For this review, take the finished solid that the model builds, in its own axes (mm). A direction names the side the tool comes from. Coordinates: 2 decimals unless noted, no trailing zeros. Loops run counter-clockwise (first coordinate to the right, second up) from the corner with the lowest first, then second, coordinate; pieces in that order, holes last. Notation, with made-up numbers: (62, 46) - (119, 46) arc R20 ccw to (119, 79) - close; hole circle Ø1 at (-38, 77.25). An arc over 180 degrees is marked (long way). Answer as a JSON object with one key per item and string values. Group by question number.
Item 1: Clearance check with flat-ended pins moving along their axes: pin 1 (1.5 mm diameter, centred on x = 0, z = -7, fed in from -Y); pin 2 (0.6 mm diameter, centred on x = 1.5, z = 1, fed in from +Y); pin 3 (1 mm diameter, centred on y = -2.5, z = -1.5, fed in from -X); pin 4 (0.6 mm diameter, centred on x = 0, y = 0, fed in from +Z). State where each tip first meets the part, or that it passes through.
Item 2: To check wall thickness, follow line 1 (Y direction, x = 0, z = -5); line 2 (X direction, y = 0.75, z = -4.75). State the ranges of each line that lie inside material, in increasing order.
Item 3: We need section A-A (z = -5.25). Give the boundary of the cut face in (x, y), then the cut area to 3 significant figures.
Item 4: Tool access review of faces 1 (the flat face through (0, 0, 0.37)), 2 (the flat face through (0, 0, -10)), 3 (the cylindrical face through (1.5, -0.07, -5.41)): name each direction out of +Z, -Z, +X, -X, +Y, -Y from which nothing blocks a thin tool from reaching the whole face with its end or side.
Autodesk Fusion 360 part; units mm, degrees
sketch "Sketch1" plane through (0, 0, 0) normal (0, 1, 0) x (1, 0, 0)
  line L0 (0, -1.9) -> (0, 10)
  line L1 (-3.15, 0) -> (-3.0363, -1.3)
  line L2 (-3.15, 0) -> (-1.399, 0)
  arc A0 (-3.0363, -1.3) -> (0, -1.9) centre (0, 6.0824) ccw
  line L3 (0, 10) -> (-1.5, 10)
  line L4 (-1.5, 10) -> (-1.5, 0.94)
  line L5 (-1.5, 0.94) -> (-1.299, 0.19)
  line L6 (-1.299, 0.19) -> (-1.299, 0.1)
  line L7 (-1.299, 0.1) -> (-1.399, 0.1) construction
  line L8 (-1.399, 0.1) -> (-1.399, 0) construction
  circle A1 centre (-1.399, 0.1) radius 0.1
  dimension "d13" = 5
  dimension "d14" = 6.3
  dimension "d15" = 0.6
  dimension "d17" = 1.3
  dimension "d18" = 3
  dimension "d19" = 10
  dimension "d20" = 9.06
  dimension "d22" = 0.75
  dimension "d23" = 15
  dimension "d24" = 0.1
  dimension "d25" = 0.1
  dimension "d26" = 0.2
revolve "Revolve1" add sketch "Sketch1" angle 360 about axis through (0, 0, 1.9) along (0, 0, -1) contours L0 L1 L2 A0 L3 L4 L5 L6 A1 makes body 1
ref_plane "WorkPlane1" through (0, 0, 1.9) normal (0, 0, 1) x (1, 0, 0)
sketch "Sketch2" plane through (0, 0, 1.9) normal (0, 0, 1) x (1, 0, 0)
  line L0 (-1.85, 0) -> (1.85, 0) construction
  line L1 (0, -1.85) -> (0, 1.85) construction
  line L2 (-0.331, 1.85) -> (0.331, 1.85)
  line L3 (0.331, 1.85) -> (0.331, 0.331)
  line L4 (0.331, 0.331) -> (1.85, 0.331)
  line L5 (1.85, 0.331) -> (1.85, -0.331)
  line L6 (1.85, -0.331) -> (0.331, -0.331)
  line L7 (0.331, -0.331) -> (0.331, -1.85)
  line L8 (0.331, -1.85) -> (-0.331, -1.85)
  line L9 (-0.331, -1.85) -> (-0.331, -0.331)
  line L10 (-0.331, -0.331) -> (-1.85, -0.331)
  line L11 (-1.85, -0.331) -> (-1.85, 0.331)
  line L12 (-1.85, 0.331) -> (-0.331, 0.331)
  line L13 (-0.331, 0.331) -> (-0.331, 1.85)
  dimension "d39" = 3.7
  dimension "d40" = 3.7
  dimension "d41" = 0.662
  dimension "d42" = 0.662
extrude "Extrude1" add sketch "Sketch2" against normal blind 1.53 separate body makes body 2
draft "Draft1" angle -30 neutral plane through (0, 0, 1.9) pull (0, 0, 1) 4 faces at (0.1103, -1.85, 1.39) (-0.1103, 1.85, 1.39) (-1.85, -0.1103, 1.39) (1.85, 0.1103, 1.39) on bodies 2
fillet "Fillet1" radius 0.662 4 edges at (0.331, -0.331, 1.135) (-0.331, -0.331, 1.135) (-0.331, 0.331, 1.135) (0.331, 0.331, 1.135) on bodies 2
combine "Combine1" operation cut target body 1 tool bodies 2
thread "Thread1"
equation "adsk_nomdia = 3.00 mm"
equation "adsk_nomlen = 10.00 mm"
equation "adsk_headdia = 6.30 mm"
equation "adsk_bheig = 1.30 mm"
equation "adsk_phildia = 3.70 mm"
equation "adsk_r = 0.10 mm"
equation "adsk_thrlen = 9.06 mm"
equation "adsk_phildepth = 1.53 mm"
equation "adsk_grplen = 0.94 mm"
equation "adsk_runout = 0.75 mm"
equation "adsk_runang = 15.00 deg"
equation "adsk_headang = 5.00 deg"
equation "d13 = adsk_headang"
equation "d14 = adsk_headdia"
equation "d15 = adsk_ovalh"
equation "adsk_ovalh = 0.60 mm"
equation "d17 = adsk_bheig"
equation "d18 = adsk_nomdia"
equation "d19 = adsk_nomlen"
equation "d20 = adsk_thrlen"
equation "d22 = adsk_runout"
equation "d24 = adsk_r"
equation "d25 = adsk_r"
equation "d26 = adsk_r * 2"
equation "d32 = adsk_bheig + adsk_ovalh"
equation "adsk_philwidth = 0.662 mm"
equation "d39 = adsk_phildia"
equation "d40 = adsk_phildia"
equation "d41 = adsk_philwidth"
equation "d42 = adsk_philwidth"
equation "d48 = adsk_philwidth"
properties part number "arrangementsContainer"
Check sheet entries:
{
 "1": {"pin 1": "stops at y = -1.5", "pin 2": "stops at y = 2.82", "pin 3": "passes through", "pin 4": "stops at z = 0.37"},
 "2": {"line 1": "y = -1.5 to 1.5", "line 2": "x = -1.3 to 1.3"},
 "3": {"outline": "circle Ø3 at (0, 0)", "area": "7.07 mm2"},
 "4": {"face 1": "+Z", "face 2": "-Z, +X, -X, +Y, -Y", "face 3": "-Z"}
}
